Autodesk Inventor part; units mm, degrees
ref_plane "YZ Plane" through (0, 0, 0) normal (1, 0, 0) x (0, 1, 0)
ref_plane "XZ Plane" through (0, 0, 0) normal (0, 1, 0) x (-1, 0, 0)
ref_plane "XY Plane" through (0, 0, 0) normal (0, 0, 1) x (1, 0, 0)
sketch "Boceto1" plane through (0, 0, 0) normal (0, 1, 0) x (-1, 0, 0)
  circle A0 centre (0, 0) radius 11
  dimension "d0" = 22
extrude "Extrusión1" add sketch "Boceto1" along normal blind 80
fillet "Empalme1" radius 10 1 edges at (11, 0, 0)
sketch "Boceto2" plane through (0, 80, 0) normal (0, 1, 0) x (1, 0, 0)
  point P0 (0, 0)
sketch "Boceto3" plane through (0, 80, 0) normal (0, 1, 0) x (1, 0, 0)
  circle A0 centre (0, 0) radius 4
  dimension "d4" = 8
extrude "Extrusión2" cut sketch "Boceto3" against normal blind 70
properties part number "pieza2 proyecto alternativo"
For this review, take the finished solid that the model builds, in its own axes (mm). Coordinates: 2 decimals unless noted, no trailing zeros. Order: outer loops, then holes, each group sorted by start corner. A loop starts at its lowest first (then second) coordinate and runs counter-clockwise, first axis right, second up. Notation, with made-up numbers: (28.25, 0.25) - (77.25, 0.25) arc R11 ccw to (77.25, 10.25) - close; hole circle Ø11 at (36, -28). An arc over 180 degrees is marked (long way). Answer as a JSON object with one key per item and string values. Group by question number.
1. The part is to be moulded in two halves that separate along X. For faces 1 (the cylindrical face through (2.38, 44.51, 10.74)), 2 (the cylindrical face through (-0.867, 45.49, 3.905)), 3 (the flat face through (0, 10, 0)), 4 (the flat face through (0, 80, -5)), say which applies: pulls with the +X half, pulls with the -X half, needs draft (parallel to the pull), parting line crosses it, or undercut.
2. Clearance check with flat-ended pins moving along their axes: P1, Ø2, axis at x = 1.5, z = 8, coming from the -Y side; P2, Ø5, axis at x = 8.5, z = 9, coming from the -Y side; P3, Ø8, axis at x = 5.5, y = 8.5, coming from the +Z side. State where each tip first meets the part, or that it passes through.
3. For probe 1 along Z at (x, y) = (0, 57); probe 2 along X at (y, z) = (74.5, 2.25); probe 3 along Z at (x, y) = (3.25, 57.5), list the stretches that pass through material, from the lowest coordinate up.
4. We need section A-A on y = 27. State the section outline as (x, z) points.
Final values:
{
 "1": {"face 1": "parting line crosses it", "face 2": "undercut", "face 3": "undercut", "face 4": "needs draft"},
 "2": {"P1": "y = 2.11", "P2": "y = 5.4", "P3": "z = 10.87"},
 "3": {"probe 1": "-11 to -4, 4 to 11", "probe 2": "-10.77 to -3.31, 3.31 to 10.77", "probe 3": "-10.51 to -2.33, 2.33 to 10.51"},
 "4": {"outline": "circle Ø22 at (0, 0); hole circle Ø8 at (0, 0)"}
}
